```python
from build123d import *

# Parameters (mm, degrees)
F0_W     = 50
F0_H     = 30
F1_DEPTH = 25
F2_R     = 10.5679387912
F3_DEPTH = 25


# Not quite as in the source:
# - a feature of the source that left no trace in its solid (it failed there, or was rolled back) is left out


with BuildPart() as f1:
    # F0 (on Front) → F1 (new body)
    with BuildSketch(Plane.XZ):
        with Locations((1.7205976233, 19.2674261052)):
            Rectangle(F0_W, F0_H)
    extrude(amount=F1_DEPTH)

    # F2 (on face) → F3 (cut)
    with BuildSketch(Plane.XZ.offset(25)):
        with Locations((-4.9288761802, 20.7236856222)):
            Circle(F2_R)
    extrude(amount=-F3_DEPTH, mode=Mode.SUBTRACT)


solid = f1.part
```
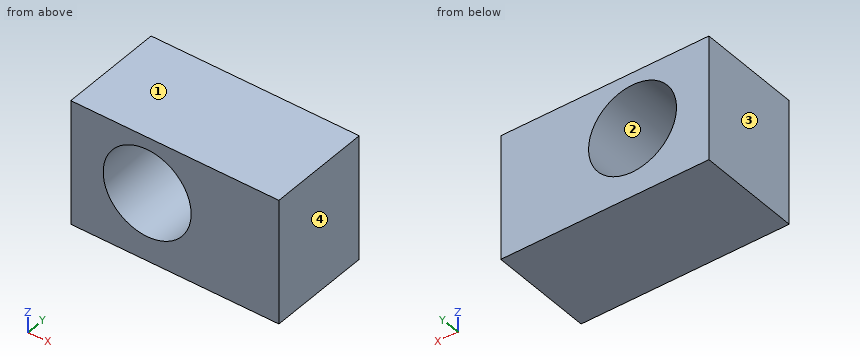
Here's how the part is built. I have some questions about the finished solid (model axes, mm). Face numbers are marked on the shaded views. Coordinates: 2 decimals unless noted, no trailing zeros. Loops run counter-clockwise (first coordinate to the right, second up) from the corner with the lowest first, then second, coordinate; pieces in that order, holes last. Notation, with made-up numbers: (59.25, 61.5) - (99.25, 61.5) arc R19 cw to (99.25, 97.5) - close; hole circle Ø9 at (27, -28). An arc over 180 degrees is marked (long way). Return JSON: item names as keys, results as strings. Group by question number.
Item 1: I need wall thicknesses on line 1 (Z direction, x = -4.5, y = -22.5); line 2 (X direction, y = -19.5, z = 19); line 3 (Z direction, x = -12.5, y = -4). Which ranges of each line are inside material? Lowest first, please. Write a range as from..to.
Item 2: If we section it at C-C on y = -15.75: Write out the boundary of the cut face in (x, z), and give its area (3 significant figures).
Item 3: Will this pin go through, and if not, where does the flat tip stop? P1, Ø12, axis at x = 1, z = 14.5, coming from the +Y side.
Item 4: We'd pull the mould along X, two halves only. Please class the marked faces 1, 2, 3 and 4: +X half, -X half, draft (parallel to the pull), parting line (faces both ways), or undercut.
Item 5: If we section it at B-B on x = -11.5: Write out the boundary of the cut face in (y, z), and give its area (3 significant figures).
Item 6: If we section it at A-A on z = 16: Write out the boundary of the cut face in (x, y).
Calculated:
{
 "1": {"line 1": "z = 4.27..10.16, 31.28..34.27", "line 2": "x = -23.28..-15.36, 5.5..26.72", "line 3": "z = 4.27..13.35, 28.1..34.27"},
 "2": {"outline": "(-23.28, 4.27) - (26.72, 4.27) - (26.72, 34.27) - (-23.28, 34.27) - close; hole circle Ø21.14 at (-4.93, 20.72)", "area": "1,150 mm^2"},
 "3": {"P1": "stops at y = 0"},
 "4": {"face 1": "draft", "face 2": "undercut", "face 3": "-X half", "face 4": "+X half"},
 "5": {"outline": "(-25, 4.27) - (0, 4.27) - (0, 12.45) - (-25, 12.45) - close; (-25, 29) - (0, 29) - (0, 34.27) - (-25, 34.27) - close", "area": "336 mm^2"},
 "6": {"outline": "(-23.28, -25) - (-14.38, -25) - (-14.38, 0) - (-23.28, 0) - close; (4.52, -25) - (26.72, -25) - (26.72, 0) - (4.52, 0) - close"}
}
